from build123d import *

# Parameters (mm, degrees)
BOSS_EXTRUDE1_DEPTH = 2
SKETCH6_R           = 10
CUT_EXTRUDE1_DEPTH  = 3


with BuildPart() as part:
    # Sketch1 → Boss-Extrude1 (new body)
    with BuildSketch(Plane(origin=(0, 0, 0), x_dir=(1, 0, 0), z_dir=(0, 1, 0))):
        with BuildLine():
            Line((-28.760538659, 18.535245878), (-28.760538659, -16.464754122))
            ThreePointArc((-28.760538659, -16.464754122), (-21.019242456, -20.723457919), (-16.760538659, -28.464754122))
            Line((-16.760538659, -28.464754122), (18.239461341, -28.464754122))
            ThreePointArc((18.239461341, -28.464754122), (22.498165139, -20.723457919), (30.239461341, -16.464754122))
            Line((30.239461341, -16.464754122), (30.239461341, 18.535245878))
            ThreePointArc((30.239461341, 18.535245878), (22.498165139, 22.793949675), (18.239461341, 30.535245878))
            Line((18.239461341, 30.535245878), (-16.760538659, 30.535245878))
            ThreePointArc((-16.760538659, 30.535245878), (-21.019242456, 22.793949675), (-28.760538659, 18.535245878))
        make_face()
    extrude(amount=BOSS_EXTRUDE1_DEPTH)

    # Sketch6 → Cut-Extrude1 (cut)
    with BuildSketch(Plane(origin=(0, 2, 0), x_dir=(1, 0, 0), z_dir=(0, 1, 0))):
        with Locations((0.739461341, 1.035245878)):
            Circle(SKETCH6_R)
    extrude(amount=-CUT_EXTRUDE1_DEPTH, mode=Mode.SUBTRACT)


solid = part.part
Work out the finished part from the listing and answer in its coordinate system (mm). Give positions to 0.01 mm unless a question says otherwise; leave off trailing zeros. Order: outer loops, then holes, each group sorted by start corner. A loop starts at its lowest first (then second) coordinate and runs counter-clockwise, first axis right, second up. Notation, with made-up numbers: (-19, -36) -> (8, -36) arc R19 cw to (8, -26) -> close; hole circle Ø4 at (66.25, 62.25). An arc over 180 degrees is marked (long way). Answer as a JSON object with one key per item and string values. Group by question number.
1. The mould has two halves that part along X. Classify faces 1 (the cylindrical face through (22.587, 0.986, -22.706)), 2 (the cylindrical face through (-20.931, 0.986, -22.883)), 3 (the cylindrical face through (-7.196, 1.014, 5.05)): released by +X, released by -X, zero draft, split by the parting line, or undercut.
2. Consider line 1 along X through (y, z) = (1.2, -1); line 2 along Z through (x, y) = (0.5, 1.05); line 3 along Z through (x, y) = (5.5, 0.4). Determine where each line is inside the solid, lowest interval first. Write a range as [from, to].
3. Section B-B on z = 0.5 is taken. Determine the outline of the cut face in (x, y), plus the area to 3 significant figures.
4. Section A-A on x = 0.5 is taken. Determine the outline of the cut face in (y, z).
5. Section D-D on z = 18 is taken. Determine the outline of the cut face in (x, y), plus the area to 3 significant figures.
6. Section C-C on y = 0.7 is taken. Determine the outline of the cut face in (x, z), plus the area to 3 significant figures.
Result sheet:
{
 "1": {"face 1": "released by +X", "face 2": "released by -X", "face 3": "undercut"},
 "2": {"line 1": "x = [-28.76, -9.26], [10.74, 30.24]", "line 2": "z = [-30.54, -11.03], [8.96, 28.46]", "line 3": "z = [-30.54, -9.83], [7.76, 28.46]"},
 "3": {"outline": "(-28.76, 0) -> (-9.14, 0) -> (-9.14, 2) -> (-28.76, 2) -> close; (10.62, 0) -> (30.24, 0) -> (30.24, 2) -> (10.62, 2) -> close", "area": "78.5 mm^2"},
 "4": {"outline": "(0, -30.54) -> (2, -30.54) -> (2, -11.03) -> (0, -11.03) -> close; (0, 8.96) -> (2, 8.96) -> (2, 28.46) -> (0, 28.46) -> close"},
 "5": {"outline": "(-24.67, 0) -> (26.15, 0) -> (26.15, 2) -> (-24.67, 2) -> close", "area": "102 mm^2"},
 "6": {"outline": "(-28.76, -18.54) arc R15.85 cw to (-16.76, -30.54) -> (18.24, -30.54) arc R15.85 cw to (30.24, -18.54) -> (30.24, 16.46) arc R15.85 cw to (18.24, 28.46) -> (-16.76, 28.46) arc R15.85 cw to (-28.76, 16.46) -> close; hole circle Ø20 at (0.74, -1.04)", "area": "2,770 mm^2"}
}
